from build123d import *

# Parameters (mm, degrees)
CROQUIS1_W                                           = 50
CROQUIS1_H                                           = 50
CROQUIS1_R                                           = 2
SALIENTE_EXTRUIR2_DEPTH                              = 100
CROQUIS4_W                                           = 3.2
CROQUIS4_H                                           = 40
SALIENTE_EXTRUIR5_DEPTH                              = 10.2
CROQUIS8_R                                           = 4
CORTAR_EXTRUIR3_DEPTH                                = 87.4
CORTAR_EXTRUIR2_START                                = -50
CROQUIS7_R                                           = 2
CORTAR_EXTRUIR2_DEPTH                                = 50
REFRENTADO_PARA_TORNILLO_TAP_N_CON_CABEZ_D           = 4.5
REFRENTADO_PARA_TORNILLO_TAP_N_CON_CABEZ_CSINK_D     = 8.96
REFRENTADO_PARA_TORNILLO_TAP_N_CON_CABEZ_CSINK_ANGLE = 90
SALIENTE_EXTRUIR6_DEPTH                              = 1.95
SALIENTE_EXTRUIR7_START                              = -5.15
SALIENTE_EXTRUIR7_DEPTH                              = 1.95
SALIENTE_EXTRUIR9_DEPTH                              = 1.95
SALIENTE_EXTRUIR10_START                             = -5.15
SALIENTE_EXTRUIR10_DEPTH                             = 1.95
SALIENTE_EXTRUIR11_START                             = -25
SALIENTE_EXTRUIR11_DEPTH                             = 5
CROQUIS17_R                                          = 2.25
CORTAR_EXTRUIR4_DEPTH                                = 2.6
REFRENTADO_PARA_TORNILLO_TAP_N_CON_C_2_D             = 4.5
REFRENTADO_PARA_TORNILLO_TAP_N_CON_C_2_CSINK_D       = 8.96
REFRENTADO_PARA_TORNILLO_TAP_N_CON_C_2_CSINK_ANGLE   = 90


with BuildPart() as part:
    # Croquis1 → Saliente-Extruir2 (new body)
    with BuildSketch(Plane.XY):
        Rectangle(CROQUIS1_W, CROQUIS1_H)
        Circle(CROQUIS1_R, mode=Mode.SUBTRACT)
    extrude(amount=SALIENTE_EXTRUIR2_DEPTH)

    # Croquis2 → Cortar-Revolución1 (revolve, cut)
    with BuildSketch(Plane(origin=(0, 0, 0), x_dir=(0, 0, -1), z_dir=(1, 0, 0))):
        Polygon((-100, 15.2), (-100, 0), (-89.8, 0), (-89.8, 10), (-97.8, 15.2), align=None)
    revolve(axis=Axis((0, 0, 100), (0, 0, -1)), mode=Mode.SUBTRACT)

    # Croquis4 → Saliente-Extruir5 (add)
    with BuildSketch(Plane.XY.offset(100)):
        with Locations((-6.6, 0)):
            Rectangle(CROQUIS4_W, CROQUIS4_H)
        with Locations((6.6, 0)):
            Rectangle(CROQUIS4_W, CROQUIS4_H)
    extrude(amount=-SALIENTE_EXTRUIR5_DEPTH)

    # Croquis8 → Cortar-Extruir3 (cut)
    with BuildSketch(Plane.XY.offset(89.8)):
        Circle(CROQUIS8_R)
    extrude(amount=-CORTAR_EXTRUIR3_DEPTH, mode=Mode.SUBTRACT)

    # Croquis7 → Cortar-Extruir2 (cut)
    with BuildSketch(Plane.ZY.offset(25).offset(CORTAR_EXTRUIR2_START)):
        with Locations((95, 0)):
            Circle(CROQUIS7_R)
    extrude(amount=CORTAR_EXTRUIR2_DEPTH, mode=Mode.SUBTRACT)

    # Refrentado para tornillo tap_n con cabez (through all)
    with Locations(Plane.ZY.offset(25)):
        with Locations((95, 0)):
            CounterSinkHole(REFRENTADO_PARA_TORNILLO_TAP_N_CON_CABEZ_D / 2, REFRENTADO_PARA_TORNILLO_TAP_N_CON_CABEZ_CSINK_D / 2, counter_sink_angle=REFRENTADO_PARA_TORNILLO_TAP_N_CON_CABEZ_CSINK_ANGLE)

    # Croquis12 → Saliente-Extruir6 (add)
    with BuildSketch(Plane.ZY.offset(25)):
        Polygon((100, 45), (80, 25), (100, 25), align=None)
    extrude(amount=-SALIENTE_EXTRUIR6_DEPTH)

    # Croquis12<2> → Saliente-Extruir7 (add)
    with BuildSketch(Plane.ZY.offset(25).offset(SALIENTE_EXTRUIR7_START)):
        Polygon((100, 45), (80, 25), (100, 25), align=None)
    extrude(amount=-SALIENTE_EXTRUIR7_DEPTH)

    # Croquis15 → Saliente-Extruir9 (add)
    with BuildSketch(Plane.XZ.offset(25)):
        Polygon((25, 100), (25, 80), (45, 100), align=None)
    extrude(amount=-SALIENTE_EXTRUIR9_DEPTH)

    # Croquis15<2> → Saliente-Extruir10 (add)
    with BuildSketch(Plane.XZ.offset(25).offset(SALIENTE_EXTRUIR10_START)):
        Polygon((25, 100), (25, 80), (45, 100), align=None)
    extrude(amount=-SALIENTE_EXTRUIR10_DEPTH)

    # Croquis16 → Saliente-Extruir11 (add, symmetric)
    with BuildSketch(Plane(origin=(25, 0, 0), x_dir=(0, 0, -1), z_dir=(1, 0, 0)).offset(SALIENTE_EXTRUIR11_START)):
        Polygon((0, 25), (-10, 25), (0, 27.6), (20, 27.6), (20, 25), align=None)
    saliente_extruir11 = extrude(amount=SALIENTE_EXTRUIR11_DEPTH, both=True)

    # Croquis17 → Cortar-Extruir4 (cut)
    with BuildSketch(Plane(origin=(0, 27.6, 0), x_dir=(1, 0, 0), z_dir=(0, 1, 0))):
        with Locations((0, 12)):
            Circle(CROQUIS17_R)
    cortar_extruir4 = extrude(amount=-CORTAR_EXTRUIR4_DEPTH, mode=Mode.SUBTRACT)

    # Refrentado para tornillo tap_n con c 2 (through all)
    with Locations(Plane(origin=(0, 27.6, 0), x_dir=(1, 0, 0), z_dir=(0, 1, 0))):
        with Locations((0, 12)):
            refrentado_para_tornillo_tap_n_con_c_2 = CounterSinkHole(REFRENTADO_PARA_TORNILLO_TAP_N_CON_C_2_D / 2, REFRENTADO_PARA_TORNILLO_TAP_N_CON_C_2_CSINK_D / 2, counter_sink_angle=REFRENTADO_PARA_TORNILLO_TAP_N_CON_C_2_CSINK_ANGLE)

    # Simetría1: Saliente-Extruir11, Cortar-Extruir4, Refrentado para tornillo tap_n con c 2 across plane
    add(saliente_extruir11.mirror(Plane(origin=(0, 0, 0), x_dir=(0, 0, 1), z_dir=(0.707106781, -0.707106781, 0))))
    add(cortar_extruir4.mirror(Plane(origin=(0, 0, 0), x_dir=(0, 0, 1), z_dir=(0.707106781, -0.707106781, 0))), mode=Mode.SUBTRACT)
    add(refrentado_para_tornillo_tap_n_con_c_2.mirror(Plane(origin=(0, 0, 0), x_dir=(0, 0, 1), z_dir=(0.707106781, -0.707106781, 0))), mode=Mode.SUBTRACT)


solid = part.part
Verification items for the finished model (mm, model axes). A direction names the side the tool comes from. Give positions to 0.01 mm unless a question says otherwise; leave off trailing zeros. Write each loop counter-clockwise with the first axis right and the second up, starting at its lowest first coordinate (ties: lowest second). Pieces come first, ordered by that corner, then holes. Notation, with made-up numbers: (35.25, 27) - (89.25, 27) arc R31 cw to (89.25, 60) - close; hole circle Ø10 at (14, -30.5). An arc over 180 degrees is marked (long way). Answer as CSV lines item,"result". Start each with the question number.
1. Sectioned sample at C-C (x = 0). Record the boundary of the cut face in (y, z), then the cut area to 3 significant figures.
2. Set-up check for faces 1 (the face through (0.09, -12.06, 92.97)), 2 (the face through (-23.05, 31, 94)), 3 (the face through (26, -5, -9)), 4 (the face through (33, -17.9, 92)), 5 (the face through (25, 1.2, -9.9)): record each of +Z, -Z, +X, -X, +Y, -Y from which the full face is reachable in a straight line by a thin tool's end or side.
3. Sectioned sample at B-B (z = 68). Record the boundary of the cut face in (x, y), then the cut area to 3 significant figures.
4. Sectioned sample at A-A (x = 23). Record the boundary of the cut face in (y, z), then the cut area to 3 significant figures.
5. Thickness scan on line 1 (Z direction, x = -16.75, y = 0); line 2 (X direction, y = -1, z = 92.5); line 3 (Y direction, x = -6, z = 95). Record the ranges inside material, lowest first.
6. Sectioned sample at D-D (y = 0). Count the separate pieces of the cut face and the enclosed holes in it, then the cut area to 3 significant figures.
7. Depth check by flat-ended pin: pin 1 (10 mm diameter, centred on x = 5, y = -7, fed in from -Z); pin 2 (5 mm diameter, centred on y = 0.5, z = -12, fed in from -X); pin 3 (5 mm diameter, centred on y = 0, z = 93.5, fed in from -X). Enter the tip coordinate at first touch or a pass-through.
8. Draft check along Z on faces 6 (the face through (-17.9, 31, 94)), 7 (the face through (-2, -1, 2.4)), 8 (the face through (-6.58, -0.86, 92.92)). Enter one of: pulls with the +Z half, pulls with the -Z half, needs draft (parallel to the pull), parting line crosses it, or undercut.
Derived:
1,outline,"(-25, 0) - (-2, 0) - (-2, 2.4) - (-4, 2.4) - (-4, 89.8) - (-10, 89.8) - (-15.2, 97.8) - (-15.2, 100) - (-25, 100) - close; (2, 0) - (25, 0) - (25, -9.75) - (25.37, -9.75) - (27.6, -7.52) - (27.6, 0) - (25, 10) - (25, 100) - (15.2, 100) - (15.2, 97.8) - (10, 89.8) - (4, 89.8) - (4, 2.4) - (2, 2.4) - close; (25, -20) - (27.6, -20) - (27.6, -16.48) - (25.37, -14.25) - (25, -14.25) - close"
1,area,"4,070 mm²"
2,face 1,"+Z"
2,face 2,"+Z, -Z, +Y"
2,face 3,"+Z, -Z, +X, -Y"
2,face 4,"+Z, -Z, +X, +Y"
2,face 5,"-Z, -X, +Y, -Y"
3,outline,"(-25, -25) - (25, -25) - (25, 25) - (-25, 25) - close; hole circle Ø8 at (0, 0)"
3,area,"2,450 mm²"
4,outline,"(-25, 0) - (25, 0) - (25, 100) - (-25, 100) - close; hole circle Ø4.5 at (0, 95)"
4,area,"4,980 mm²"
5,line 1,"0 to 92.75, 97.25 to 100"
5,line 2,"-23.21 to -11.71, -8.2 to -5, 5 to 8.2, 11.71 to 25"
5,line 3,"-25 to -2.25, 2.25 to 25"
6,separate pieces,"7"
6,enclosed holes,"0"
6,area,"4,000 mm²"
7,pin 1,"z = 0"
7,pin 2,"x = 25"
7,pin 3,"x = -24.52"
8,face 6,"needs draft"
8,face 7,"pulls with the +Z half"
8,face 8,"undercut"
